Can you work these out from the model? Positions are in its coordinate system, mm. A direction names the side the tool comes from. Coordinates: 2 decimals unless noted, no trailing zeros. Order: outer loops, then holes, each group sorted by start corner. A loop starts at its lowest first (then second) coordinate and runs counter-clockwise, first axis right, second up.
```python
from build123d import *

# Parameters (mm, degrees)
SKETCH_1_W               = 52
SKETCH_1_H               = 33.6
EXTRUDE_1_DEPTH          = 5
SKETCH_3_R               = 3
CUT_EXTRUDE_2_DEPTH      = 5
SKETCH_4_R               = 9.3
EXTRUDE_2_DEPTH          = 11
CUT_EXTRUDE_3_DEPTH      = 11
CUT_EXTRUDE_3_DEPTH_BACK = 11
SKETCH_5_R               = 1.5


with BuildPart() as part:
    # 草图1 → 凸台-拉伸1 (new body)
    with BuildSketch(Plane.XY):
        Rectangle(SKETCH_1_W, SKETCH_1_H)
    extrude(amount=EXTRUDE_1_DEPTH)

    # 草图3 → 切除-拉伸2 (cut)
    with BuildSketch(Plane.XY.offset(5)):
        with Locations((-20, 11)):
            Circle(SKETCH_3_R)
        with Locations((20, -11)):
            Circle(SKETCH_3_R)
    extrude(amount=-CUT_EXTRUDE_2_DEPTH, mode=Mode.SUBTRACT)

    # 草图4 → 凸台-拉伸2 (add)
    with BuildSketch(Plane.XY.offset(5)):
        with Locations(Location((0, 0, 0), (0, 0, 180))):
            Circle(SKETCH_4_R)
        with BuildLine():
            Line((3.166622807, -4.25), (-3.166622807, -4.25))
            ThreePointArc((-3.166622807, -4.25), (0, 5.3), (3.166622807, -4.25))
        make_face(mode=Mode.SUBTRACT)
    extrude(amount=EXTRUDE_2_DEPTH)

    # 草图5 → 切除-拉伸3 (cut, two sides: drawn at the far end of the back side and taken through both)
    with BuildSketch(Plane(origin=(0, 0, 0), x_dir=(1, 0, 0), z_dir=(0, 1, 0)).offset(-CUT_EXTRUDE_3_DEPTH_BACK)):
        with Locations(Location((0, -13, 0), (0, 0, 90))):
            Circle(SKETCH_5_R)
    extrude(amount=CUT_EXTRUDE_3_DEPTH + CUT_EXTRUDE_3_DEPTH_BACK, mode=Mode.SUBTRACT)


solid = part.part
```
1. Imagine slicing it at A-A on x = 0. Please give me the cut outline in (y, z), then the cut area to 3 significant figures.
Completed:
outline: (-16.8, 0) - (16.8, 0) - (16.8, 5) - (9.3, 5) - (9.3, 11.5) - (5.3, 11.5) - (5.3, 5) - (-4.25, 5) - (-4.25, 11.5) - (-9.3, 11.5) - (-9.3, 5) - (-16.8, 5) - close; (-9.3, 14.5) - (-4.25, 14.5) - (-4.25, 16) - (-9.3, 16) - close; (5.3, 14.5) - (9.3, 14.5) - (9.3, 16) - (5.3, 16) - close
area: 240 mm2
2. Please list where these lines run through material, in increasing order: probe 1 along Y at (x, z) = (-20, 3.15); probe 2 along Z at (x, y) = (-15.5, -11.5); probe 3 along X at (y, z) = (8.5, 14).
Completed:
probe 1: y = -16.8 to 8, 14 to 16.8
probe 2: z = 0 to 5
probe 3: x = -3.77 to -1.12, 1.12 to 3.77
3. On a 3-axis mill with a long thin cutter (end or side, diameter ignored), from which of +Z, -Z, +X, -X, +Y, -Y can I reach the whole of each face in a straight line? I mean faces 1 (the cylindrical face through (-4.29, 8.25, 10.42)), 2 (the cylindrical face through (-0.07, -6.81, 14.5)). Say none if no direction works.
Completed:
face 1: +Z
face 2: +Y, -Y
4. Imagine slicing it at D-D on y = 11. Please give me the cut outline in (x, z).
Completed:
outline: (-26, 0) - (-23, 0) - (-23, 5) - (-26, 5) - close; (-17, 0) - (26, 0) - (26, 5) - (-17, 5) - close
5. Thinking about a two-plate mould opening in Y: for faces 3 (the cylindrical face through (17, -11, 3)), 4 (the flat face through (26, 0, 2)), 5 (the flat face through (0, -16.8, 2)), which applies, pulls with the +Y half, pulls with the -Y half, needs draft (parallel to the pull), parting line crosses it, or undercut?
Completed:
face 3: undercut
face 4: needs draft
face 5: pulls with the -Y half
6. Imagine slicing it at C-C on x = 20. Please give me the cut outline in (y, z), then the cut area to 3 significant figures.
Completed:
outline: (-16.8, 0) - (-14, 0) - (-14, 5) - (-16.8, 5) - close; (-8, 0) - (16.8, 0) - (16.8, 5) - (-8, 5) - close
area: 138 mm2
7. Imagine slicing it at B-B on z = 2. Please give me the cut outline in (x, y), then the cut area to 3 significant figures.
Completed:
outline: (-26, -16.8) - (26, -16.8) - (26, 16.8) - (-26, 16.8) - close; hole circle Ø6 at (-20, 11); hole circle Ø6 at (20, -11)
area: 1,690 mm2
8. I'm going to push flat-ended pins straight in: pin 1 (1.5 mm diameter, centred on x = -9.5, y = -6, fed in from +Z); pin 2 (3.5 mm diameter, centred on x = 0, z = 13, fed in from -Y); pin 3 (2 mm diameter, centred on x = 7.5, z = 7.5, fed in from +Y); pin 4 (6 mm diameter, centred on x = -7, z = 6.5, fed in from +Y). Where does each tip first touch, or does it pass through?
Completed:
pin 1: stops at z = 5
pin 2: stops at y = -9.3
pin 3: stops at y = 6.65
pin 4: stops at y = 16.8
